Check sheet for the drawn part. Datum: minimum x, y, z corner. Units: mm. Coordinates: 2 decimals unless noted, no trailing zeros. Write each loop counter-clockwise with the first axis right and the second up, starting at its lowest first coordinate (ties: lowest second). Pieces come first, ordered by that corner, then holes. Notation, with made-up numbers: (45, -9.75) - (91, -9.75) arc R23 ccw to (91, 25.25) - close; hole circle Ø7 at (42.25, 82). An arc over 180 degrees is marked (long way). Use one line per item in the form item = value. Start each with the question number.
1. Cross-section at C-C on y = 9. Record the boundary of the cut face in (x, z), then the cut area to 3 significant figures.
2. Scan lines: line 1 along X through (y, z) = (3.75, 6); line 2 along Z through (x, y) = (100.5, 7.5); line 3 along X through (y, z) = (9, 51). Record each from-to range of solid material in increasing order.
3. Draft check along Y on the marked faces 1 and 2. Enter one of: +Y half, -Y half, draft (parallel to the pull), parting line (faces both ways), or undercut.
4. Cross-section at A-A on x = 177. Record the boundary of the cut face in (y, z), then the cut area to 3 significant figures.
5. Cross-section at B-B on z = 63.5. Record the boundary of the cut face in (x, y).
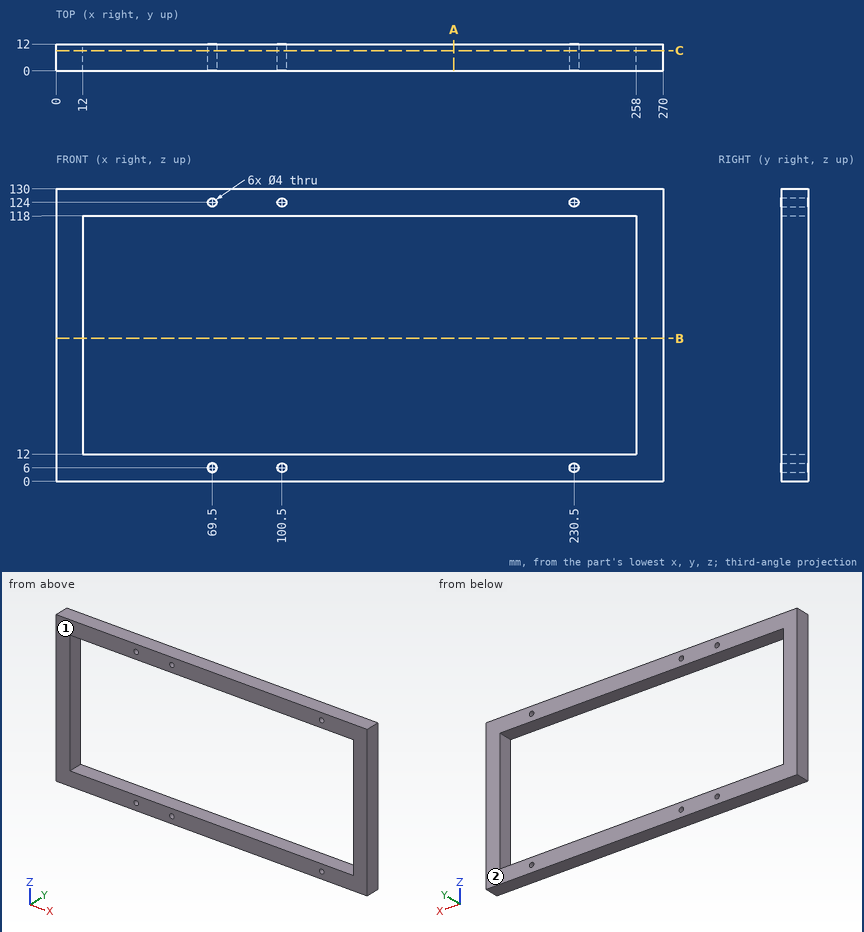
Final values:
q1.outline = (0, 0) - (270, 0) - (270, 130) - (0, 130) - close; hole (12, 12) - (258, 12) - (258, 118) - (12, 118) - close; hole circle Ø4 at (69.5, 6); hole circle Ø4 at (69.5, 124); hole circle Ø4 at (100.5, 6); hole circle Ø4 at (100.5, 124); hole circle Ø4 at (230.5, 6); hole circle Ø4 at (230.5, 124)
q1.area = 8,950 mm²
q2.line_1 = 0 to 67.5, 71.5 to 98.5, 102.5 to 228.5, 232.5 to 270
q2.line_2 = 0 to 4, 8 to 12, 118 to 122, 126 to 130
q2.line_3 = 0 to 12, 258 to 270
q3.face_1 = -Y half
q3.face_2 = +Y half
q4.outline = (0, 0) - (12, 0) - (12, 12) - (0, 12) - close; (0, 118) - (12, 118) - (12, 130) - (0, 130) - close
q4.area = 288 mm²
q5.outline = (0, 0) - (12, 0) - (12, 12) - (0, 12) - close; (258, 0) - (270, 0) - (270, 12) - (258, 12) - close
